Work out the finished part from the listing and answer in its coordinate system (mm). Face numbers are marked on the shaded views. A direction names the side the tool comes from. Round coordinates to 2 decimals unless told otherwise and drop trailing zeros. Order: outer loops, then holes, each group sorted by start corner. A loop starts at its lowest first (then second) coordinate and runs counter-clockwise, first axis right, second up. Notation, with made-up numbers: (4, 10.5) -> (31, 10.5) arc R25 cw to (31, 42.5) -> close; hole circle Ø6 at (-28, 24). An arc over 180 degrees is marked (long way). Use a Markdown table: item, result. Add a question column.
Item 1: For a pull along Y with two mould halves and no side action, classify the marked faces 1, 2 and 3 as +Y half, -Y half, draft (parallel to the pull), parting line (faces both ways), or undercut.
Item 2: A cutting plane is placed at C-C, the plane x = 0. Determine the outline of the cut face in (y, z).
Item 3: Flat-ended cylindrical pins translate along their axes: P1, Ø5, axis at x = -49.5, y = 55.5, coming from the +Z side; P2, Ø1, axis at x = 53, z = 234, coming from the -Y side; P3, Ø3, axis at x = -74, y = 27, coming from the +Z side. Find the tip coordinate at first contact, or state that the pin passes through.
Item 4: A cutting plane is placed at B-B, the plane x = 24. Determine the outline of the cut face in (y, z), plus the area to 3 significant figures.
Item 5: A tool of negligible diameter and unlimited length cuts with its end or side. For the marked faces 4 and 5, from which of +Z, -Z, +X, -X, +Y, -Y can it reach the whole face along a straight path? Write none if from no direction.
Item 6: Find the intervals of material crossed by L1, parallel to Y at x = -60.5, z = 64.5; L2, parallel to X at y = 30, z = 172; L3, parallel to Z at x = -24, y = 15.5, in increasing order. Write a range as [from, to].
Item 7: A cutting plane is placed at D-D, the plane y = 47. Determine the outline of the cut face in (x, z), plus the area to 3 significant figures.
Item 8: A cutting plane is placed at A-A, the plane z = 78. Determine the outline of the cut face in (x, y).
from build123d import *

# Parameters (mm, degrees)
F0_W         = 150.5279913545
F0_H         = 149.8499512672
F1_DEPTH     = 194.6834623814
F2_T         = -2.54
F3_W         = 2.54
F3_H         = 2.54
F4_DEPTH     = 95.1251834631
F6_D         = 101.6
F6_DEPTH     = 2.541
F7_T1_DEPTH  = 202.3034623814
F7_T3_DEPTH  = 297.4286458445
F7_T5_DEPTH  = 140.3679913545
F7_T7_DEPTH  = 139.6899512672
F7_T9_DEPTH  = 175.9279913545
F7_S13_W     = 5.08
F7_S13_H     = 5.08
F7_T14_DEPTH = 5.08
F7_S19_W     = 5.08
F7_S19_H     = 5.08
F7_T20_DEPTH = 5.08
F7_S25_W     = 5.08
F7_S25_H     = 5.08
F7_T26_DEPTH = 5.08
F7_S31_W     = 5.08
F7_S31_H     = 5.08
F7_T32_DEPTH = 5.08
F8_W         = 145.4479913545
F8_H         = 10.8655169606
F9_DEPTH     = 192.7349418402
F11_D        = 25.4
F11_DEPTH    = 12.7
F11_TIP      = 7.6309298617


# Not quite as in the source:
# - a fillet or chamfer that OpenCascade refuses, or shapes differently, is made with other operations: its cross-section is extruded or revolved along the edge and cut away or added


with BuildPart() as f1:
    # F0 (on Top) → F1 (new body)
    with BuildSketch(Plane.XY):
        with Locations((-0.0158064067, 0.4480481148)):
            Rectangle(F0_W, F0_H)
    extrude(amount=F1_DEPTH)

    # F2
    f2_openings = [f1.faces().sort_by_distance(p)[0] for p in [
        (-0.015806, 0.448048, 194.683462),
    ]]
    offset(amount=F2_T, openings=f2_openings)

    # F3 (on face) → F4 (join)
    with BuildSketch(Plane.XY.offset(194.6834623814)):
        Polygon((72.7081892705, 75.3730237484), (-75.279802084, 75.3730237484), (-75.279802084, 72.8330237484), (-72.739802084, 72.8330237484), (72.7081892705, 72.8330237484), align=None)
        with Locations((73.9781892705, 74.1030237484)):
            Rectangle(F3_W, F3_H)
    extrude(amount=F4_DEPTH)

    # F6 (through all, one way)
    with BuildSketch(Plane.XZ.offset(-72.8330237484)):
        with Locations((0, 236.040353775)):
            Circle(F6_D / 2)
    extrude(amount=-F6_DEPTH, mode=Mode.SUBTRACT)

    # F7: fillet of radius 5.08 on 9 edges, made by hand

    # F7_s2 → F7_t1 (cut)
    with BuildSketch(Plane.XY.offset(5.08)):
        with BuildLine():
            ThreePointArc((-75.279802084, -69.3969275188), (-73.7919045324, -72.9890299673), (-70.199802084, -74.4769275188))
            Line((-70.199802084, -74.4769275188), (-75.279802084, -74.4769275188))
            Line((-75.279802084, -74.4769275188), (-75.279802084, -69.3969275188))
        make_face()
        with BuildLine():
            ThreePointArc((75.2481892705, -69.3969275188), (73.7602917189, -72.9890299673), (70.1681892705, -74.4769275188))
            Line((70.1681892705, -74.4769275188), (75.2481892705, -74.4769275188))
            Line((75.2481892705, -74.4769275188), (75.2481892705, -69.3969275188))
        make_face()
    extrude(amount=F7_T1_DEPTH, mode=Mode.SUBTRACT)

    # F7_s4 → F7_t3 (cut)
    with BuildSketch(Plane.XY.offset(5.08)):
        with BuildLine():
            ThreePointArc((-70.199802084, 75.3730237484), (-73.7919045324, 73.8851261968), (-75.279802084, 70.2930237484))
            Line((-75.279802084, 70.2930237484), (-75.279802084, 75.3730237484))
            Line((-75.279802084, 75.3730237484), (-70.199802084, 75.3730237484))
        make_face()
        with BuildLine():
            ThreePointArc((70.1681892705, 75.3730237484), (73.7602917189, 73.8851261968), (75.2481892705, 70.2930237484))
            Line((75.2481892705, 70.2930237484), (75.2481892705, 75.3730237484))
            Line((75.2481892705, 75.3730237484), (70.1681892705, 75.3730237484))
        make_face()
    extrude(amount=F7_T3_DEPTH, mode=Mode.SUBTRACT)

    # F7_s6 → F7_t5 (cut)
    with BuildSketch(Plane.YZ.offset(-70.199802084)):
        with BuildLine():
            ThreePointArc((75.3730237484, 5.08), (73.8851261968, 1.4878975516), (70.2930237484, 0))
            Line((70.2930237484, 0), (75.3730237484, 0))
            Line((75.3730237484, 0), (75.3730237484, 5.08))
        make_face()
        with BuildLine():
            ThreePointArc((-69.3969275188, 0), (-72.9890299673, 1.4878975516), (-74.4769275188, 5.08))
            Line((-74.4769275188, 5.08), (-74.4769275188, 0))
            Line((-74.4769275188, 0), (-69.3969275188, 0))
        make_face()
    extrude(amount=F7_T5_DEPTH, mode=Mode.SUBTRACT)

    # F7_s8 → F7_t7 (cut)
    with BuildSketch(Plane.XZ.offset(-70.2930237484)):
        with BuildLine():
            ThreePointArc((-70.199802084, 0), (-73.7919045324, 1.4878975516), (-75.279802084, 5.08))
            Line((-75.279802084, 5.08), (-75.279802084, 0))
            Line((-75.279802084, 0), (-70.199802084, 0))
        make_face()
        with BuildLine():
            ThreePointArc((75.2481892705, 5.08), (73.7602917189, 1.4878975516), (70.1681892705, 0))
            Line((70.1681892705, 0), (75.2481892705, 0))
            Line((75.2481892705, 0), (75.2481892705, 5.08))
        make_face()
    extrude(amount=F7_T7_DEPTH, mode=Mode.SUBTRACT)

    # F7_s10 → F7_t9 (cut)
    with BuildSketch(Plane.YZ.offset(-87.979802084)):
        with BuildLine():
            ThreePointArc((-74.4769275188, 189.6034623814), (-72.9890299673, 193.1955648298), (-69.3969275188, 194.6834623814))
            Line((-69.3969275188, 194.6834623814), (-74.4769275188, 194.6834623814))
            Line((-74.4769275188, 194.6834623814), (-74.4769275188, 189.6034623814))
        make_face()
    extrude(amount=F7_T9_DEPTH, mode=Mode.SUBTRACT)


with BuildPart() as f7_tool12:
    # F7_s13 → F7_t14 (new body)
    with BuildSketch(Plane.XY.offset(5.08)):
        with Locations((-72.739802084, -71.9369275188)):
            Rectangle(F7_S13_W, F7_S13_H)
    extrude(amount=-F7_T14_DEPTH)

    # F7_s15 → F7_t16 (revolve, cut)
    with BuildSketch(Plane(origin=(-70.199802084, -69.3969275188, 5.08), x_dir=(0.7071067812, 0.7071067812, 0), z_dir=(-0.7071067812, 0.7071067812, 0))):
        with BuildLine():
            ThreePointArc((0, -5.08), (5.08, 0), (0, 5.08))
            Line((0, 5.08), (0, -5.08))
        make_face()
    revolve(axis=Axis((-70.199802084, -69.3969275188, 5.08), (0, 0, -1)), mode=Mode.SUBTRACT)


with BuildPart() as f1_1:
    add(f1.part)

    # F7_t11: cut F7_tool12
    add(f7_tool12.part, mode=Mode.SUBTRACT)


with BuildPart() as f7_tool18:
    # F7_s19 → F7_t20 (new body)
    with BuildSketch(Plane.XZ.offset(-70.2930237484)):
        with Locations((-72.739802084, 2.54)):
            Rectangle(F7_S19_W, F7_S19_H)
    extrude(amount=-F7_T20_DEPTH)

    # F7_s21 → F7_t22 (revolve, cut)
    with BuildSketch(Plane(origin=(-70.199802084, 70.2930237484, 5.08), x_dir=(0.7071067812, 0, 0.7071067812), z_dir=(-0.7071067812, 0, 0.7071067812))):
        with BuildLine():
            ThreePointArc((0, -5.08), (5.08, 0), (0, 5.08))
            Line((0, 5.08), (0, -5.08))
        make_face()
    revolve(axis=Axis((-70.199802084, 70.2930237484, 5.08), (0, 1, 0)), mode=Mode.SUBTRACT)


with BuildPart() as f1_2:
    add(f1_1.part)

    # F7_t17: cut F7_tool18
    add(f7_tool18.part, mode=Mode.SUBTRACT)


with BuildPart() as f7_tool24:
    # F7_s25 → F7_t26 (new body)
    with BuildSketch(Plane.XZ.offset(-70.2930237484)):
        with Locations((72.7081892705, 2.54)):
            Rectangle(F7_S25_W, F7_S25_H)
    extrude(amount=-F7_T26_DEPTH)

    # F7_s27 → F7_t28 (revolve, cut)
    with BuildSketch(Plane(origin=(70.1681892705, 70.2930237484, 5.08), x_dir=(-0.7071067812, 0, 0.7071067812), z_dir=(-0.7071067812, 0, -0.7071067812))):
        with BuildLine():
            ThreePointArc((0, -5.08), (5.08, 0), (0, 5.08))
            Line((0, 5.08), (0, -5.08))
        make_face()
    revolve(axis=Axis((70.1681892705, 70.2930237484, 5.08), (0, 1, 0)), mode=Mode.SUBTRACT)


with BuildPart() as f1_3:
    add(f1_2.part)

    # F7_t23: cut F7_tool24
    add(f7_tool24.part, mode=Mode.SUBTRACT)


with BuildPart() as f7_tool30:
    # F7_s31 → F7_t32 (new body)
    with BuildSketch(Plane.YZ.offset(70.1681892705)):
        with Locations((-71.9369275188, 2.54)):
            Rectangle(F7_S31_W, F7_S31_H)
    extrude(amount=F7_T32_DEPTH)

    # F7_s33 → F7_t34 (revolve, cut)
    with BuildSketch(Plane(origin=(70.1681892705, -69.3969275188, 5.08), x_dir=(0, 0.7071067812, 0.7071067812), z_dir=(0, 0.7071067812, -0.7071067812))):
        with BuildLine():
            ThreePointArc((0, -5.08), (5.08, 0), (0, 5.08))
            Line((0, 5.08), (0, -5.08))
        make_face()
    revolve(axis=Axis((70.1681892705, -69.3969275188, 5.08), (1, 0, 0)), mode=Mode.SUBTRACT)


with BuildPart() as f1_4:
    add(f1_3.part)

    # F7_t29: cut F7_tool30
    add(f7_tool30.part, mode=Mode.SUBTRACT)

    # F8 (on face) → F9 (join)
    with BuildSketch(Plane.XY.offset(2.54)):
        with Locations((-0.0158064067, -21.8428857625)):
            Rectangle(F8_W, F8_H)
    extrude(amount=F9_DEPTH)

    # F11 (one way)
    with BuildSketch(Plane.XZ.offset(27.2756442428)):
        with Locations((-4.689078778, 137.1918618679)):
            Circle(F11_D / 2)
    extrude(amount=-F11_DEPTH, mode=Mode.SUBTRACT)
    with Locations(Plane.XZ.offset(27.2756442428)):
        with Locations((-4.689078778, 137.1918618679)):
            with Locations((0, 0, -(F11_DEPTH + F11_TIP / 2))):  # 118° drill point
                Cone(0, F11_D / 2, F11_TIP, mode=Mode.SUBTRACT)


solid = f1_4.part
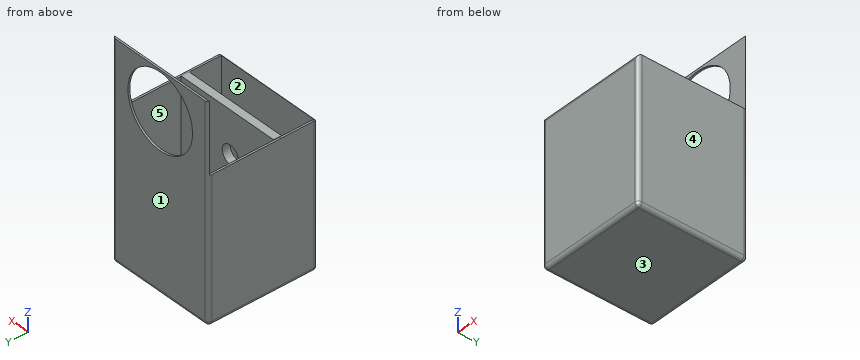
Reported:
| question | item | result |
|---|---|---|
| 1 | face 1 | +Y half |
| 1 | face 2 | undercut |
| 1 | face 3 | draft |
| 2 | outline | (-74.48, 5.08) arc R5.08 ccw to (-69.4, 0) -> (70.29, 0) arc R5.08 ccw to (75.37, 5.08) -> (75.37, 185.24) -> (72.83, 185.24) -> (72.83, 2.54) -> (-16.41, 2.54) -> (-16.41, 125.39) -> (-27.28, 125.39) -> (-27.28, 2.54) -> (-71.94, 2.54) -> (-71.94, 194) arc R5.08 ccw to (-74.48, 189.6) -> close; (-27.28, 148.99) -> (-16.41, 148.99) -> (-16.41, 195.27) -> (-27.28, 195.27) -> close; (72.83, 286.84) -> (75.37, 286.84) -> (75.37, 289.81) -> (72.83, 289.81) -> close |
| 3 | P1 | z = 2.54 |
| 3 | P2 | y = 72.83 |
| 3 | P3 | z = 194.68 |
| 4 | outline | (-74.48, 5.08) arc R5.08 ccw to (-69.4, 0) -> (70.29, 0) arc R5.08 ccw to (75.37, 5.08) -> (75.37, 191.27) -> (72.83, 191.27) -> (72.83, 2.54) -> (-16.41, 2.54) -> (-16.41, 195.27) -> (-27.28, 195.27) -> (-27.28, 2.54) -> (-71.94, 2.54) -> (-71.94, 194) arc R5.08 ccw to (-74.48, 189.6) -> close; (72.83, 280.81) -> (75.37, 280.81) -> (75.37, 289.81) -> (72.83, 289.81) -> close |
| 4 | area | 3,450 mm² |
| 5 | face 4 | +Z, -Z, +X, +Y, -Y |
| 5 | face 5 | +Z |
| 6 | L1 | [-74.48, -71.94], [-27.28, -16.41], [72.83, 75.37] |
| 6 | L2 | [-75.28, -72.74], [72.71, 75.25] |
| 6 | L3 | [0, 2.54] |
| 7 | outline | (-75.28, 5.08) arc R5.08 ccw to (-70.2, 0) -> (70.17, 0) arc R5.08 ccw to (75.25, 5.08) -> (75.25, 194.68) -> (72.71, 194.68) -> (72.71, 2.54) -> (-72.74, 2.54) -> (-72.74, 194.68) -> (-75.28, 194.68) -> close |
| 7 | area | 1,350 mm² |
| 8 | outline | (-75.28, -69.4) arc R5.08 ccw to (-70.2, -74.48) -> (70.17, -74.48) arc R5.08 ccw to (75.25, -69.4) -> (75.25, 70.29) arc R5.08 ccw to (70.17, 75.37) -> (-70.2, 75.37) arc R5.08 ccw to (-75.28, 70.29) -> close; hole (-72.74, -71.94) -> (72.71, -71.94) -> (72.71, -27.28) -> (-72.74, -27.28) -> close; hole (-72.74, -16.41) -> (72.71, -16.41) -> (72.71, 72.83) -> (-72.74, 72.83) -> close |
